Geometry: final body of the model. Coordinates: model frame, mm. A direction names the side the tool comes from. Coordinates: 2 decimals unless noted, no trailing zeros. Order: outer loops, then holes, each group sorted by start corner. A loop starts at its lowest first (then second) coordinate and runs counter-clockwise, first axis right, second up. Notation, with made-up numbers: (10.5, 83) -> (66.5, 83) arc R8 ccw to (66.5, 92) -> close; hole circle Ø2 at (-8, 86.5). An arc over 180 degrees is marked (long way). Use one line per item in the form item = value.
```python
from build123d import *

# Parameters (mm, degrees)
BOSS_EXTRUDE1_DEPTH        = 5
F_3_2_3_2_DIAMETER_HOLE1_D = 3.2
BOSS_EXTRUDE2_DEPTH        = 5
SKETCH10_W                 = 7
SKETCH10_H                 = 7
CUT_EXTRUDE2_DEPTH         = 2.6
SKETCH11_R                 = 2.1
CUT_EXTRUDE3_DEPTH         = 41.33014714


with BuildPart() as part:
    # Sketch1 → Boss-Extrude1 (new body)
    with BuildSketch(Plane(origin=(0, 0, 0), x_dir=(1, 0, 0), z_dir=(0, 1, 0))):
        with BuildLine():
            Line((-216.657705663, 38.202599087), (-206.809628133, 36.46611731))
            ThreePointArc((-206.809628133, 36.46611731), (-210, 0), (-206.809628133, -36.46611731))
            Line((-206.809628133, -36.46611731), (-216.657705663, -38.202599087))
            ThreePointArc((-216.657705663, -38.202599087), (-220, 0), (-216.657705663, 38.202599087))
        make_face()
    extrude(amount=BOSS_EXTRUDE1_DEPTH)

    # Ø3.2 (3.2) Diameter Hole1 (through all)
    with Locations(Plane(origin=(0, 0, 0), x_dir=(-1, 0, 0), z_dir=(0, -1, 0))):
        with Locations((214.18186009, -18.738484691), (214.18186009, 18.738484691), (213.160645195, -28.063131327), (213.160645195, 28.063131327)):
            Hole(F_3_2_3_2_DIAMETER_HOLE1_D / 2)

    # Sketch9 → Boss-Extrude2 (add)
    with BuildSketch(Plane(origin=(0, 5, 0), x_dir=(1, 0, 0), z_dir=(0, 1, 0))):
        with BuildLine():
            Line((-219.772609758, 10), (-209.761769634, 10))
            ThreePointArc((-209.761769634, 10), (-210, 0), (-209.761769634, -10))
            Line((-209.761769634, -10), (-219.772609758, -10))
            ThreePointArc((-219.772609758, -10), (-220, 0), (-219.772609758, 10))
        make_face()
    extrude(amount=BOSS_EXTRUDE2_DEPTH)

    # Sketch10 → Cut-Extrude2 (cut)
    with BuildSketch(Plane.ZY.offset(215)):
        with Locations((0, 10)):
            Rectangle(SKETCH10_W, SKETCH10_H)
    extrude(amount=-CUT_EXTRUDE2_DEPTH, mode=Mode.SUBTRACT)

    # Sketch11 → Cut-Extrude3 (cut, through all)
    with BuildSketch(Plane.ZY.offset(215)):
        with Locations((0, 10)):
            Circle(SKETCH11_R)
    extrude(amount=-CUT_EXTRUDE3_DEPTH, mode=Mode.SUBTRACT)


solid = part.part
```
1) Material intervals for probe 1 along Y at (x, z) = (-212, 34.5); probe 2 along X at (y, z) = (3, -1); probe 3 along Z at (x, y) = (-215, 6), sorted ascending. Write a range as from..to.
Results found:
probe_1 = 0..5
probe_2 = -220..-210
probe_3 = -10..10
2) Section A-A, the plane y = 4.25. Output: boundary loops of the cut face in (x, z), and give its area (3 significant figures).
Results found:
outline = (-216.66, -38.2) -> (-206.81, -36.47) arc R210 cw to (-206.81, 36.47) -> (-216.66, 38.2) arc R220 ccw to start; hole circle Ø3.2 at (-214.18, -18.74); hole circle Ø3.2 at (-214.18, 18.74); hole circle Ø3.2 at (-213.16, -28.06); hole circle Ø3.2 at (-213.16, 28.06)
area = 718 mm2
3) Pull-direction query (X, two-part tool) for faces 5 (the flat face through (-213, 0, -1)), 6 (the cylindrical face through (-211.635, 2.535, 27.583)), 7 (the flat face through (-211.803, 2.465, -37.347)); classes: released by +X, released by -X, zero draft, split by the parting line, or undercut.
Results found:
face_5 = zero draft
face_6 = undercut
face_7 = released by +X
4) Access query for faces 1 (the flat face through (-215, 7, 10)), 2 (the flat face through (-214, 8, -3.5)), 3 (the flat face through (-215, 7, -10)), 4 (the cylindrical face through (-211.2, 7.9, 0)). Directions: +Z, -Z, +X, -X, +Y, -Y. A direction counts if a zero-diameter tool reaches every point of the face in a straight line with its end or side. Return the directions, or none.
Results found:
face_1 = +Z, +X, -X, +Y
face_2 = +Y
face_3 = -Z, +X, -X, +Y
face_4 = +X, +Y
5) Section D-D, the plane z = 31. Output: boundary loops of the cut face in (x, y).
Results found:
outline = (-217.8, 0) -> (-207.7, 0) -> (-207.7, 5) -> (-217.8, 5) -> close
6) Contact query for flat-ended pins moving along their axis: P1, Ø3, axis at x = -213.16, z = 28.06, coming from the +Y side; P2, Ø5.5, axis at x = -213, y = 8, coming from the +Z side; P3, Ø1.3, axis at x = -214, z = 0, coming from the +Y side; P4, Ø3, axis at x = -210.5, y = 7.5, coming from the -Z side. Output: stop coordinate, or through.
Results found:
P1 = through
P2 = 10
P3 = 6.5
P4 = -10
7) Section B-B, the plane z = 0. Output: boundary loops of the cut face in (x, y).
Results found:
outline = (-220, 0) -> (-210, 0) -> (-210, 7.9) -> (-212.4, 7.9) -> (-212.4, 6.5) -> (-215, 6.5) -> (-215, 10) -> (-220, 10) -> close
